Answer from the drawing. Dimensions are ordinates in mm from the lowest x, y and z of the part. A direction names the side the tool comes from. Round coordinates to 2 decimals unless told otherwise and drop trailing zeros. Loops run counter-clockwise (first coordinate to the right, second up) from the corner with the lowest first, then second, coordinate; pieces in that order, holes last.
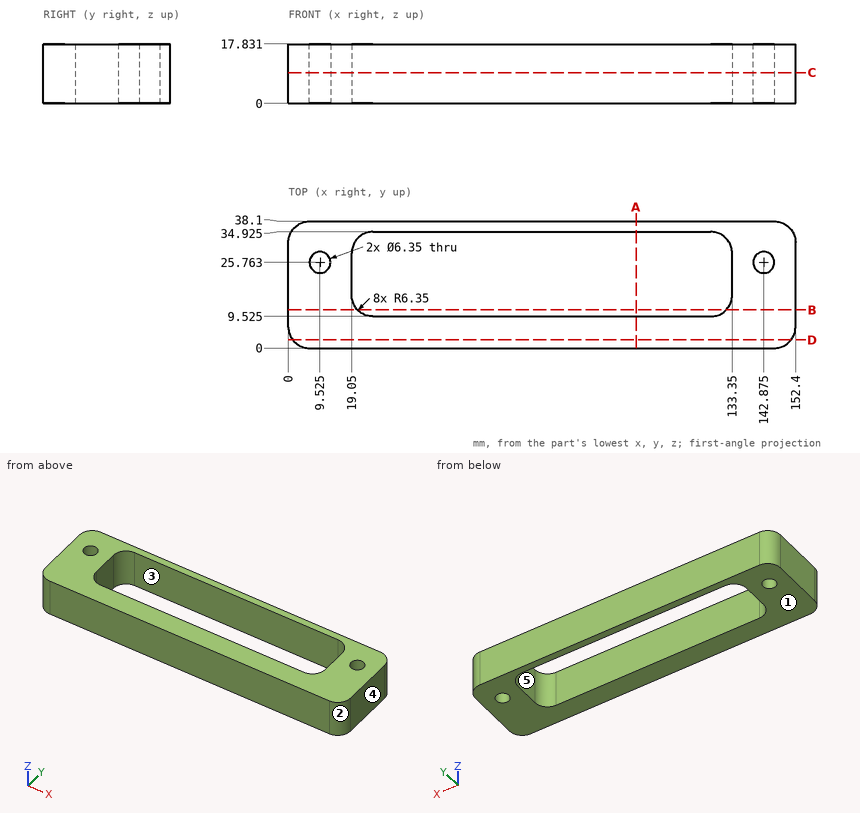
1. Which of the six approach directions +Z, -Z, +X, -X, +Y, -Y give full straight-line access (tool end or side, diameter ignored) to the marked faces 4 and 5?
Answer key:
face 4: +Z, -Z, +X, +Y, -Y
face 5: +Z, -Z
2. Find section C-C (z = 9.25). Write down the section's boundary in (x, y) (3 decimals).
Answer key:
outline: (0, 6.35) arc R6.35 ccw to (6.35, 0) - (146.05, 0) arc R6.35 ccw to (152.4, 6.35) - (152.4, 31.75) arc R6.35 ccw to (146.05, 38.1) - (6.35, 38.1) arc R6.35 ccw to (0, 31.75) - close; hole circle Ø6.35 at (9.525, 25.763); hole (19.05, 15.875) arc R6.35 ccw to (25.4, 9.525) - (127, 9.525) arc R6.35 ccw to (133.35, 15.875) - (133.35, 28.575) arc R6.35 ccw to (127, 34.925) - (25.4, 34.925) arc R6.35 ccw to (19.05, 28.575) - close; hole circle Ø6.35 at (142.875, 25.763)
3. Find section B-B (y = 11.5). Write down the section's boundary in (x, z), then the cut area to 3 significant figures.
Answer key:
outline: (0, 0) - (20.8, 0) - (20.8, 17.83) - (0, 17.83) - close; (131.6, 0) - (152.4, 0) - (152.4, 17.83) - (131.6, 17.83) - close
area: 742 mm2
4. Find section A-A (x = 104.5). Write down the section's boundary in (y, z) (1 decimal), then the cut area to 3 significant figures.
Answer key:
outline: (0, 0) - (9.5, 0) - (9.5, 17.8) - (0, 17.8) - close; (34.9, 0) - (38.1, 0) - (38.1, 17.8) - (34.9, 17.8) - close
area: 226 mm2
5. Find section D-D (y = 2.5). Write down the section's boundary in (x, z).
Answer key:
outline: (1.3, 0) - (151.1, 0) - (151.1, 17.83) - (1.3, 17.83) - close
6. Consider probe 1 along X at (y, z) = (26, 5); probe 2 along Y at (x, z) = (108.5, 17.25) (3 decimals); probe 3 along X at (y, z) = (18.5, 17). Determine where each line is inside the solid, lowest interval first.
Answer key:
probe 1: x = 0 to 6.36, 12.69 to 19.05, 133.35 to 139.71, 146.04 to 152.4
probe 2: y = 0 to 9.525, 34.925 to 38.1
probe 3: x = 0 to 19.05, 133.35 to 152.4
7. Determine the mould class of the marked faces 1, 2 and 3 for opening direction X: +X half, -X half, draft (parallel to the pull), parting line (faces both ways), or undercut.
Answer key:
face 1: draft
face 2: +X half
face 3: undercut
